Verification items for the finished model (mm, model axes). A direction names the side the tool comes from. Give positions to 0.01 mm unless a question says otherwise; leave off trailing zeros. Write each loop counter-clockwise with the first axis right and the second up, starting at its lowest first coordinate (ties: lowest second). Pieces come first, ordered by that corner, then holes. Notation, with made-up numbers: M 7.5,-24.5 L 43.5,-24.5 A25 cw 43.5,-8.5 Z; hole C 89,79.5 d11. An arc over 180 degrees is marked long. Write item = value, one per line.
from build123d import *

# Parameters (mm, degrees)
SKETCH_1_W          = 20
SKETCH_1_H          = 20
SKETCH_1_W_2        = 18
SKETCH_1_H_2        = 18
EXTRUDE_1_DEPTH     = 650
SKETCH_3_R          = 1.6
CUT_EXTRUDE_1_DEPTH = 651.38450166
SKETCH_4_R          = 1.6
CUT_EXTRUDE_2_DEPTH = 651.38450166
SKETCH_5_R          = 1.55
CUT_EXTRUDE_3_DEPTH = 651.38450166


with BuildPart() as part:
    # 草图1 → 拉伸-薄壁1 (new body)
    with BuildSketch(Plane(origin=(0, 0, 0), x_dir=(1, 0, 0), z_dir=(0, 1, 0))):
        Rectangle(SKETCH_1_W, SKETCH_1_H)
        Rectangle(SKETCH_1_W_2, SKETCH_1_H_2, mode=Mode.SUBTRACT)
    extrude(amount=EXTRUDE_1_DEPTH)

    # 草图3 → 切除-拉伸1 (cut, through all)
    with BuildSketch(Plane(origin=(10, 0, 0), x_dir=(0, 0, -1), z_dir=(1, 0, 0))):
        with Locations((-5, 15)):
            Circle(SKETCH_3_R)
        with Locations((-5, 5)):
            Circle(SKETCH_3_R)
        with Locations((5, 5)):
            Circle(SKETCH_3_R)
        with Locations((5, 15)):
            Circle(SKETCH_3_R)
        with Locations((5, 635)):
            Circle(SKETCH_3_R)
        with Locations((5, 645)):
            Circle(SKETCH_3_R)
        with Locations((-5, 645)):
            Circle(SKETCH_3_R)
        with Locations((-5, 635)):
            Circle(SKETCH_3_R)
    extrude(amount=-CUT_EXTRUDE_1_DEPTH, mode=Mode.SUBTRACT)

    # 草图4 → 切除-拉伸2 (cut, through all)
    with BuildSketch(Plane.XY.offset(10)):
        with Locations((0, 35)):
            Circle(SKETCH_4_R)
        with Locations((0, 55)):
            Circle(SKETCH_4_R)
        with Locations((0, 75)):
            Circle(SKETCH_4_R)
        with Locations((0, 95)):
            Circle(SKETCH_4_R)
        with Locations((0, 115)):
            Circle(SKETCH_4_R)
        with Locations((0, 135)):
            Circle(SKETCH_4_R)
        with Locations((0, 155)):
            Circle(SKETCH_4_R)
        with Locations((0, 175)):
            Circle(SKETCH_4_R)
        with Locations((0, 195)):
            Circle(SKETCH_4_R)
        with Locations((0, 215)):
            Circle(SKETCH_4_R)
        with Locations((0, 235)):
            Circle(SKETCH_4_R)
        with Locations((0, 255)):
            Circle(SKETCH_4_R)
        with Locations((0, 275)):
            Circle(SKETCH_4_R)
        with Locations((0, 295)):
            Circle(SKETCH_4_R)
        with Locations((0, 315)):
            Circle(SKETCH_4_R)
        with Locations((0, 335)):
            Circle(SKETCH_4_R)
        with Locations((0, 355)):
            Circle(SKETCH_4_R)
        with Locations((0, 375)):
            Circle(SKETCH_4_R)
        with Locations((0, 395)):
            Circle(SKETCH_4_R)
        with Locations((0, 415)):
            Circle(SKETCH_4_R)
        with Locations((0, 435)):
            Circle(SKETCH_4_R)
        with Locations((0, 455)):
            Circle(SKETCH_4_R)
        with Locations((0, 475)):
            Circle(SKETCH_4_R)
        with Locations((0, 495)):
            Circle(SKETCH_4_R)
        with Locations((0, 515)):
            Circle(SKETCH_4_R)
        with Locations((0, 535)):
            Circle(SKETCH_4_R)
        with Locations((0, 555)):
            Circle(SKETCH_4_R)
        with Locations((0, 575)):
            Circle(SKETCH_4_R)
        with Locations((0, 595)):
            Circle(SKETCH_4_R)
        with Locations((0, 615)):
            Circle(SKETCH_4_R)
    extrude(amount=-CUT_EXTRUDE_2_DEPTH, mode=Mode.SUBTRACT)

    # 草图5 → 切除-拉伸3 (cut, through all)
    with BuildSketch(Plane.XY.offset(10)):
        with Locations((-5, 15)):
            Circle(SKETCH_5_R)
        with Locations(Location((-5, 5, 0), (0, 0, 180))):
            Circle(SKETCH_5_R)
        with Locations((5, 5)):
            Circle(SKETCH_5_R)
        with Locations(Location((5, 15, 0), (0, 0, 180))):
            Circle(SKETCH_5_R)
    extrude(amount=-CUT_EXTRUDE_3_DEPTH, mode=Mode.SUBTRACT)


solid = part.part
1) Material ranges on probe 1 along Z at (x, y) = (9.4, 645); probe 2 along Y at (x, z) = (-9.45, -5); probe 3 along Z at (x, y) = (7, 301), recorded low to high. Write a range as from..to.
From the geometry:
probe_1 = -10..-6.6, -3.4..3.4, 6.6..10
probe_2 = 0..3.4, 6.6..13.4, 16.6..633.4, 636.6..643.4, 646.6..650
probe_3 = -10..-9, 9..10
2) Tool access check on faces 5 (the flat face through (-0.8, 650, 9.6)), 6 (the flat face through (0, 320, 9)). Record the directions out of +Z, -Z, +X, -X, +Y, -Y that give a thin tool (end or side, any length) a straight path to the whole face; none if there is none.
From the geometry:
face_5 = +Z, -Z, +X, -X, +Y
face_6 = +Y, -Y
3) Draft check along Z on faces 1 (the flat face through (-0.8, 0, 9.6)), 2 (the flat face through (0, 320, -9)), 3 (the flat face through (9, 320, 0)), 4 (the flat face through (0, 320, 10)). Enter one of: +Z half, -Z half, draft (parallel to the pull), parting line (faces both ways), or undercut.
From the geometry:
face_1 = draft
face_2 = undercut
face_3 = undercut
face_4 = +Z half
4) Cross-section at A-A on y = 368. Record the boundary of the cut face in (x, z), plus the area to 3 significant figures.
From the geometry:
outline = M -10,-10 L 10,-10 L 10,10 L -10,10 Z; hole M -9,-9 L 9,-9 L 9,9 L -9,9 Z
area = 76.0 mm^2
